Part model, mm, in its own coordinate system. A direction names the side the tool comes from. Give positions to 0.01 mm unless a question says otherwise; leave off trailing zeros. Order: outer loops, then holes, each group sorted by start corner. A loop starts at its lowest first (then second) coordinate and runs counter-clockwise, first axis right, second up. Notation, with made-up numbers: (66.25, 64) - (123.25, 64) arc R19 cw to (123.25, 70) - close; hole circle Ø1 at (1, 8). An arc over 180 degrees is marked (long way). Use one line per item in the form item = value. Start each with the question number.
1. Pull direction X, two halves, no side cores. Call faces 1 (the face through (17.907, 5, 26)), 2 (the face through (33.5, 141.4, -27.9)), 3 (the face through (-21.88, 7.56, 27.5)): +X half, -X half, draft (parallel to the pull), parting line (faces both ways), or undercut.
2. Band-saw the part on B-B, the plane z = -16. List the corners of the cut face in (x, y) (3 decimals), plus the area to 3 significant figures.
3. Band-saw the part on D-D, the plane y = 20. List the corners of the cut face in (x, z) (3 decimals).
4. Band-saw the part on A-A, the plane x = -5. List the corners of the cut face in (y, z) (3 decimals).
5. Pin check, flat tips, straight feed: P1, Ø1, axis at x = 13, z = -23, coming from the +Y side (3 decimals); P2, Ø13.5, axis at x = 25.5, z = 12, coming from the +Y side (3 decimals); P3, Ø3.5, axis at x = 4.5, y = 1.5, coming from the +Z side. Stop position of each tip, or through.
6. Band-saw the part on C-C, the plane z = 25.5. List the corners of the cut face in (x, y) (3 decimals).
7. Tool access for faces 4 (the face through (5, 2, 21.5)), 5 (the face through (35, 18, -9)), 6 (the face through (-28, 13.175, 18)), 7 (the face through (-27.34, 69.58, -27.89)), 8 (the face through (0, 2, 17)): list every direction of +Z, -Z, +X, -X, +Y, -Y with a clear straight run to the whole face (end or side of a thin tool).
8. Drill centre lines: line 1 (Y direction, x = -25, z = -28.8) (3 decimals); line 2 (Y direction, x = 24.75, z = 25.5) (3 decimals); line 3 (Z direction, x = 25, y = 76) (3 decimals). Where is each one in solid material? Low to high.
from build123d import *

# Parameters (mm, degrees)
SKETCH1_W               = 70
SKETCH1_H               = 59
BOSS_EXTRUDE1_DEPTH     = 3.175
SKETCH2_W               = 70
SKETCH2_H               = 3.175
BOSS_EXTRUDE2_DEPTH     = 139.7
SKETCH4_W               = 7.5
SKETCH4_H               = 8
BOSS_EXTRUDE3_DEPTH     = 10
SKETCH5_W               = 26.289
SKETCH5_H               = 8
CUT_EXTRUDE2_DEPTH      = 10
SKETCH3_R               = 3.175
CUT_EXTRUDE1_DEPTH      = 139.7
SKETCH9_W               = 9.593
SKETCH9_H               = 55.825
BOSS_EXTRUDE4_DEPTH     = 10
SKETCH7_W               = 22
SKETCH7_H               = 27.5
CUT_EXTRUDE6_DEPTH      = 10
CUT_EXTRUDE7_DEPTH      = 153.202212694
CUT_EXTRUDE7_DEPTH_BACK = 153.202212694
SKETCH12_R              = 2
BOSS_EXTRUDE5_DEPTH     = 9.593
BOSS_EXTRUDE6_DEPTH     = 9.593
FILLET1_R               = 5.08
FILLET2_R               = 5.08
FILLET3_R               = 5.08


with BuildPart() as part:
    # Sketch1 → Boss-Extrude1 (new body)
    with BuildSketch(Plane(origin=(0, 0, 0), x_dir=(1, 0, 0), z_dir=(0, 1, 0))):
        Rectangle(SKETCH1_W, SKETCH1_H)
    extrude(amount=BOSS_EXTRUDE1_DEPTH)

    # Sketch2 → Boss-Extrude2 (add)
    with BuildSketch(Plane(origin=(0, 3.175, 0), x_dir=(1, 0, 0), z_dir=(0, 1, 0))):
        with Locations((0, 27.9125)):
            Rectangle(SKETCH2_W, SKETCH2_H)
    extrude(amount=BOSS_EXTRUDE2_DEPTH)

    # Sketch4 → Boss-Extrude3 (add)
    with BuildSketch(Plane(origin=(0, 3.175, 0), x_dir=(1, 0, 0), z_dir=(0, 1, 0))):
        with Locations((-12.132, -25.5)):
            Rectangle(SKETCH4_W, SKETCH4_H)
        with Locations((21.657, -25.5)):
            Rectangle(SKETCH4_W, SKETCH4_H)
    extrude(amount=BOSS_EXTRUDE3_DEPTH)

    # Sketch5 → Cut-Extrude2 (cut)
    with BuildSketch(Plane(origin=(0, 3.175, 0), x_dir=(1, 0, 0), z_dir=(0, 1, 0))):
        with Locations((4.7625, -25.5)):
            Rectangle(SKETCH5_W, SKETCH5_H)
    extrude(amount=-CUT_EXTRUDE2_DEPTH, mode=Mode.SUBTRACT)

    # Sketch3 → Cut-Extrude1 (cut)
    with BuildSketch(Plane.XY.offset(-26.325)):
        with Locations((-25, 136.525)):
            Circle(SKETCH3_R)
        with Locations((25.038, 136.525)):
            Circle(SKETCH3_R)
        with Locations((25.038, 67.437)):
            Circle(SKETCH3_R)
        with Locations((-25, 67.437)):
            Circle(SKETCH3_R)
    extrude(amount=-CUT_EXTRUDE1_DEPTH, mode=Mode.SUBTRACT)

    # Sketch9 → Boss-Extrude4 (add)
    with BuildSketch(Plane(origin=(0, 3.175, 0), x_dir=(1, 0, 0), z_dir=(0, 1, 0))):
        with Locations((30.2035, -1.5875)):
            Rectangle(SKETCH9_W, SKETCH9_H)
        Polygon((-25.407, 26.325), (-35, 26.325), (-35, -29.5), (-25.407, -29.5), (-15.882, -29.5), (-15.882, -21.5), (-25.407, -21.5), align=None)
    extrude(amount=BOSS_EXTRUDE4_DEPTH)

    # Sketch7 → Cut-Extrude6 (cut)
    with BuildSketch(Plane(origin=(0, 3.175, 0), x_dir=(1, 0, 0), z_dir=(0, 1, 0))):
        with Locations((0, -3.25)):
            Rectangle(SKETCH7_W, SKETCH7_H)
    extrude(amount=-CUT_EXTRUDE6_DEPTH, mode=Mode.SUBTRACT)

    # Sketch12 → Cut-Extrude7 (cut, two sides: drawn at the far end of the back side and taken through both)
    with BuildSketch(Plane(origin=(-8.382, 0, 0), x_dir=(0, 0, -1), z_dir=(1, 0, 0)).offset(-CUT_EXTRUDE7_DEPTH_BACK)):
        with Locations((-25.5, 7.475)):
            Circle(SKETCH12_R)
    extrude(amount=CUT_EXTRUDE7_DEPTH + CUT_EXTRUDE7_DEPTH_BACK, mode=Mode.SUBTRACT)

    # Sketch13 → Boss-Extrude5 (add)
    with BuildSketch(Plane.ZY.offset(35)):
        Polygon((-26.325, 13.175), (-26.325, 38.575), (-0.925, 13.175), align=None)
    extrude(amount=-BOSS_EXTRUDE5_DEPTH)

    # Sketch14 → Boss-Extrude6 (add)
    with BuildSketch(Plane(origin=(35, 0, 0), x_dir=(0, 0, -1), z_dir=(1, 0, 0))):
        Polygon((26.325, 13.175), (26.325, 38.575), (0.925, 13.175), align=None)
    extrude(amount=-BOSS_EXTRUDE6_DEPTH)

    # Fillet1
    fillet1_edges = [part.edges().sort_by_distance(p)[0] for p in [
        (-35, 142.875, -27.9125),
        (35, 142.875, -27.9125),
    ]]
    fillet(fillet1_edges, radius=FILLET1_R)

    # Fillet2
    fillet2_edges = [part.edges().sort_by_distance(p)[0] for p in [
        (-30.2035, 13.175, -0.925),
        (-30.2035, 38.575, -26.325),
        (30.2035, 13.175, -0.925),
        (30.2035, 38.575, -26.325),
    ]]
    fillet(fillet2_edges, radius=FILLET2_R)

    # Fillet3
    fillet3_edges = [part.edges().sort_by_distance(p)[0] for p in [
        (-25.407, 8.175, 21.5),
        (25.407, 8.175, 21.5),
    ]]
    fillet(fillet3_edges, radius=FILLET3_R)


solid = part.part
From the geometry:
q1.face_1 = undercut
q1.face_2 = +X half
q1.face_3 = draft
q2.outline = (-35, 0) - (35, 0) - (35, 28.25) - (25.407, 28.25) - (25.407, 3.175) - (-25.407, 3.175) - (-25.407, 28.25) - (-35, 28.25) - close
q2.area = 703 mm²
q3.outline = (-35, -29.5) - (35, -29.5) - (35, -7.75) - (25.407, -7.75) - (25.407, -26.325) - (-25.407, -26.325) - (-25.407, -7.75) - (-35, -7.75) - close
q4.outline = (0, -29.5) - (142.875, -29.5) - (142.875, -26.325) - (3.175, -26.325) - (3.175, -10.5) - (0, -10.5) - close; (0, 17) - (3.175, 17) - (3.175, 21.5) - (0, 21.5) - close
q5.P1 = 3.175
q5.P2 = 13.175
q5.P3 = 21.5
q6.outline = (-35, 0) - (-8.382, 0) - (-8.382, 5.475) - (-35, 5.475) - close; (-35, 9.475) - (-8.382, 9.475) - (-8.382, 13.175) - (-35, 13.175) - close; (17.907, 0) - (35, 0) - (35, 5.475) - (17.907, 5.475) - close; (17.907, 9.475) - (35, 9.475) - (35, 13.175) - (17.907, 13.175) - close
q7.face_4 = +Z, +Y, -Y
q7.face_5 = +Z, -Z, +X, +Y, -Y
q7.face_6 = +Z, +X, -X, +Y
q7.face_7 = +Z, -Z
q7.face_8 = +Y, -Y
q8.line_1 = 0 to 64.262, 70.612 to 133.35, 139.7 to 142.875
q8.line_2 = 0 to 5.475, 9.475 to 13.175
q8.line_3 = -29.5 to -26.325
